from build123d import *

# Parameters (mm, degrees)
SKETCH_1_R          = 5
SKETCH_1_R_2        = 2
EXTRUDE_1_DEPTH     = 12
SKETCH_2_W          = 10
SKETCH_2_H          = 17.5
EXTRUDE_2_DEPTH     = 12
SKETCH_3_R          = 2
CUT_EXTRUDE_1_DEPTH = 22.800229357
SKETCH_5_W          = 6.3
SKETCH_5_H          = 2.5
CUT_EXTRUDE_3_DEPTH = 8.48
SKETCH_10_W         = 9.65653404
SKETCH_10_H         = 7.55
CUT_EXTRUDE_5_DEPTH = 9.4
CUT_EXTRUDE_4_REACH = 27.986
SKETCH_6_R          = 1.55


with BuildPart() as part:
    # Эскиз1 → Бобышка-Вытянуть1 (new body)
    with BuildSketch(Plane.XY):
        Circle(SKETCH_1_R)
        Circle(SKETCH_1_R_2, mode=Mode.SUBTRACT)
    extrude(amount=EXTRUDE_1_DEPTH)

    # Эскиз2 → Бобышка-Вытянуть2 (add)
    with BuildSketch(Plane.XY.offset(12)):
        with Locations((0, 8.75)):
            Rectangle(SKETCH_2_W, SKETCH_2_H)
    extrude(amount=-EXTRUDE_2_DEPTH)

    # Эскиз3 → Вырез-Вытянуть1 (cut, through all)
    with BuildSketch(Plane.XY.offset(12)):
        Circle(SKETCH_3_R)
    extrude(amount=-CUT_EXTRUDE_1_DEPTH, mode=Mode.SUBTRACT)

    # Эскиз5 → Вырез-Вытянуть3 (cut)
    with BuildSketch(Plane.XY.offset(12)):
        with Locations((0.1, 14)):
            Rectangle(SKETCH_5_W, SKETCH_5_H)
    extrude(amount=-CUT_EXTRUDE_3_DEPTH, mode=Mode.SUBTRACT)

    # Эскиз10 → Вырез-Вытянуть5 (cut)
    with BuildSketch(Plane.ZY.offset(5)):
        with Locations((6.27, 6.7)):
            Rectangle(SKETCH_10_W, SKETCH_10_H)
    extrude(amount=-CUT_EXTRUDE_5_DEPTH, mode=Mode.SUBTRACT)

    # Вырез-Вытянуть4: up to this face of the body (flat: up to its plane)
    cut_extrude_4_end = Plane(part.part.faces().sort_by_distance((-0.3, 10.475, 6.27))[0])
    # Эскиз6 → Вырез-Вытянуть4 (cut, up to the picked face)
    with BuildSketch(Plane(origin=(0, 17.5, 0), x_dir=(1, 0, 0), z_dir=(0, 1, 0)), mode=Mode.PRIVATE) as cut_extrude_4_sk1:
        with Locations(Location((0, -6.27, 0), (0, 0, 270))):
            Circle(SKETCH_6_R)
    cut_extrude_4_tool1 = split(extrude(cut_extrude_4_sk1.sketch, amount=-CUT_EXTRUDE_4_REACH, mode=Mode.PRIVATE), bisect_by=cut_extrude_4_end, keep=Keep.BOTH, mode=Mode.PRIVATE)
    add(cut_extrude_4_tool1.solids().sort_by(Axis((0, 17.5, 6.27), (0, -1, 0)))[0], mode=Mode.SUBTRACT)


solid = part.part
Input: part model. Units: mm. Frame: model coordinates. A direction names the side the tool comes from. Round coordinates to 2 decimals unless told otherwise and drop trailing zeros. Loops run counter-clockwise (first coordinate to the right, second up) from the corner with the lowest first, then second, coordinate; pieces in that order, holes last. Notation, with made-up numbers: M 43.5,53 L 87.5,53 A22 ccw 87.5,78 Z; hole C 9.25,15.5 d3. An arc over 180 degrees is marked long. Answer as CSV lines item,"result". Start each with the question number.
(1) Reachability of faces 1 (the flat face through (0, 12.75, 8)), 2 (the flat face through (0, 7, 11.098)), 3 (the cylindrical face through (0.466, 16.391, 7.748)) from +Z, -Z, +X, -X, +Y, -Y: full face, straight path, thin tool, end or side. Return the list, or none.
(2) Section A-A, the plane x = 0. Output: boundary loops of the cut face in (y, z) (3 decimals).
(3) Line query: line 1 (Z direction, x = 3, y = 3); line 2 (X direction, y = 0, z = 7.25); line 3 (X direction, y = 15, z = 7). Output: solid intervals per line, ascending. Write a range as [from, to].
(4) Section C-C, the plane x = 4. Output: boundary loops of the cut face in (y, z) (3 decimals).
(5) Section D-D, the plane y = -1.5. Output: boundary loops of the cut face in (x, z).
(6) Draft query along Z for faces 4 (the flat face through (3.25, 14, 8)), 5 (the flat face through (0, 7, 1.442)), 6 (the flat face through (0, 6, 0)). Return one class per face: released by +Z, released by -Z, zero draft, split by the parting line, or undercut.
(7) Section B-B, the plane z = 6.27. Output: boundary loops of the cut face in (x, y) (3 decimals).
(8) First-contact query: pin 1 (2.5 mm diameter, centred on x = 0, y = 0, fed in from +Z); pin 2 (3 mm diameter, centred on x = 0, z = 6.27, fed in from +Y) (3 decimals); pin 3 (0.8 mm diameter, centred on x = 1.5, y = 13.5, fed in from +Z); pin 4 (3 mm diameter, centred on x = 3, z = 9.5, fed in from -Y). Flat tips, straight axial feed; report the tip coordinate or a pass-through.
Values found:
1,face 1,"+Z"
1,face 2,"-X"
1,face 3,"+Y"
2,outline,"M -5,0 L -2,0 L -2,12 L -5,12 Z; M 2,0 L 17.5,0 L 17.5,4.72 L 15.25,4.72 L 15.25,3.52 L 12.75,3.52 L 12.75,4.72 L 10.475,4.72 L 10.475,1.442 L 2.925,1.442 L 2.925,11.098 L 10.475,11.098 L 10.475,7.82 L 12.75,7.82 L 12.75,12 L 2,12 Z; M 15.25,7.82 L 17.5,7.82 L 17.5,12 L 15.25,12 Z"
3,line 1,"z = [0, 1.44], [11.1, 12]"
3,line 2,"x = [-5, -2], [2, 5]"
3,line 3,"x = [-5, -3.05], [3.25, 5]"
4,outline,"M -3,0 L 17.5,0 L 17.5,12 L -3,12 Z; hole M 2.925,1.442 L 10.475,1.442 L 10.475,11.098 L 2.925,11.098 Z"
5,outline,"M -4.77,0 L -1.32,0 L -1.32,12 L -4.77,12 Z; M 1.32,0 L 4.77,0 L 4.77,12 L 1.32,12 Z"
6,face 4,"zero draft"
6,face 5,"undercut"
6,face 6,"released by -Z"
7,outline,"M -5,0 A5 ccw 5,0 L 5,17.5 L 1.55,17.5 L 1.55,15.25 L 3.25,15.25 L 3.25,12.75 L 1.55,12.75 L 1.55,10.475 L 4.4,10.475 L 4.4,2.925 L -5,2.925 Z; M -5,10.475 L -1.55,10.475 L -1.55,12.75 L -3.05,12.75 L -3.05,15.25 L -1.55,15.25 L -1.55,17.5 L -5,17.5 Z; hole C 0,0 d4"
8,pin 1,"passes through"
8,pin 2,"stops at y = 2.925"
8,pin 3,"stops at z = 3.52"
8,pin 4,"stops at y = -4.77"
